Here's how the part is built. I have some questions about the finished solid (model axes, mm). Give positions to 0.01 mm unless a question says otherwise; leave off trailing zeros. Loops run counter-clockwise (first coordinate to the right, second up) from the corner with the lowest first, then second, coordinate; pieces in that order, holes last.
Q1. I'm going to push flat-ended pins straight in: P1, Ø5, axis at x = 81.5, z = 31, coming from the -Y side; P2, Ø8, axis at x = 22.5, y = -34, coming from the -Z side; P3, Ø8, axis at x = 86, y = -18, coming from the +Z side. Where does each tip first touch, or does it pass through?
Q2. I need wall thicknesses on probe 1 along X at (y, z) = (-5.5, 40); probe 2 along X at (y, z) = (-10.5, 32); probe 3 along X at (y, z) = (-2.5, 58). Which ranges of each line are inside material? Lowest first, please.
Q3. Suppose I cut it at D-D (x = 144). List the corners of the cut face in (y, z) for me.
Q4. Thinking about a two-plate mould opening in Z: for faces 1 (the face through (148, -50.8, 24)), 2 (the face through (99.35, -41.14, 39.4)), 3 (the face through (-53.17, -25.04, 13.87)), which applies, pulls with the +Z half, pulls with the -Z half, needs draft (parallel to the pull), parting line crosses it, or undercut?
Q5. Suppose I cut it at C-C (z = 44.5). List the corners of the cut face in (x, y) for me.
Q6. Suppose I cut it at B-B (y = -9.5). List the corners of the cut face in (x, z) for me (1 decimal).
Q7. Suppose I cut it at A-A (y = -35). List the corners of the cut face in (x, z) for me (1 decimal).
```python
from build123d import *
from build123d import SkipClean  # not in build123d's __all__

# Parameters (mm, degrees)
F0_R     = 17.4625
F1_DEPTH = 31.75
F2_DEPTH = 31.75
F0_R_2   = 25.4
F3_DEPTH = 50.8
F4_DEPTH = 12.7
F5_DEPTH = 50.8


with BuildPart() as f1:
    # F0 (on Front) → F1 (new body)
    with BuildSketch(Plane.XZ):
        with BuildLine():
            ThreePointArc((137.8952277792, 72.3404701197), (134.9898494581, 72.609247784), (132.0721238048, 72.6277311095))
            Line((132.0721238048, 72.6277311095), (137.8952277792, 72.3404701197))
        make_face()
        with BuildLine():
            Line((137.8952277792, 5.0155493856), (132.0808217973, 4.7279708331))
            ThreePointArc((132.0808217973, 4.7279708331), (134.9941960526, 4.7469864233), (137.8952277792, 5.0155493856))
        make_face()
        with BuildLine():
            Line((137.8952277792, 72.3404701197), (132.0721238048, 72.6277311095))
            ThreePointArc((132.0721238048, 72.6277311095), (99.3434793984, 38.6736578588), (132.0808217973, 4.7279708331))
            Line((132.0808217973, 4.7279708331), (137.8952277792, 5.0155493856))
            ThreePointArc((137.8952277792, 5.0155493856), (158.9060092226, 16.333410504), (167.2884791197, 38.6780097526))
            ThreePointArc((167.2884791197, 38.6780097526), (158.9060092226, 61.0226090013), (137.8952277792, 72.3404701197))
        make_face()
        with Locations((133.3159791197, 38.6780097526)):
            Circle(F0_R, mode=Mode.SUBTRACT)
    extrude(amount=F1_DEPTH)

    # F0 (on Front) → F2 (join)
    with BuildSketch(Plane.XZ):
        with BuildLine():
            ThreePointArc((-42.8278144375, 81.2557634421), (-15.6881628684, 67.2156297522), (-4.7965205083, 38.6664061547))
            ThreePointArc((-4.7965205083, 38.6664061547), (-15.6881628684, 10.1171825573), (-42.8278144375, -3.9229511326))
            Line((-42.8278144375, -3.9229511326), (132.0808217973, 4.7279708331))
            ThreePointArc((132.0808217973, 4.7279708331), (99.3434793984, 38.6736578588), (132.0721238048, 72.6277311095))
            Line((132.0721238048, 72.6277311095), (-42.8278144375, 81.2557634421))
        make_face()
    extrude(amount=F2_DEPTH)

    # F0 (on Front) → F3 (join)
    with BuildSketch(Plane.XZ):
        with BuildLine():
            ThreePointArc((-42.8278144375, -3.9229511326), (-15.6881628684, 10.1171825573), (-4.7965205083, 38.6664061547))
            ThreePointArc((-4.7965205083, 38.6664061547), (-15.6881628684, 67.2156297522), (-42.8278144375, 81.2557634421))
            ThreePointArc((-42.8278144375, 81.2557634421), (-90.5215205083, 38.6664061547), (-42.8278144375, -3.9229511326))
        make_face()
        with Locations((-47.6590205083, 38.6664061547)):
            Circle(F0_R_2, mode=Mode.SUBTRACT)
    extrude(amount=F3_DEPTH)

    # F0 (on Front) → F4 (cut)
    with BuildSketch(Plane.XZ):
        with BuildLine():
            ThreePointArc((-42.8278144375, 81.2557634421), (-15.6881628684, 67.2156297522), (-4.7965205083, 38.6664061547))
            ThreePointArc((-4.7965205083, 38.6664061547), (-15.6881628684, 10.1171825573), (-42.8278144375, -3.9229511326))
            Line((-42.8278144375, -3.9229511326), (132.0808217973, 4.7279708331))
            ThreePointArc((132.0808217973, 4.7279708331), (99.3434793984, 38.6736578588), (132.0721238048, 72.6277311095))
            Line((132.0721238048, 72.6277311095), (-42.8278144375, 81.2557634421))
        make_face()
    with SkipClean():  # cleaning this boolean's faces spoils the solid; the shape is the same uncleaned
        extrude(amount=F4_DEPTH, mode=Mode.SUBTRACT)

    # F0 (on Front) → F5 (join)
    with BuildSketch(Plane.XZ):
        with BuildLine():
            Line((137.8952277792, 72.3404701197), (132.0721238048, 72.6277311095))
            ThreePointArc((132.0721238048, 72.6277311095), (99.3434793984, 38.6736578588), (132.0808217973, 4.7279708331))
            Line((132.0808217973, 4.7279708331), (137.8952277792, 5.0155493856))
            ThreePointArc((137.8952277792, 5.0155493856), (158.9060092226, 16.333410504), (167.2884791197, 38.6780097526))
            ThreePointArc((167.2884791197, 38.6780097526), (158.9060092226, 61.0226090013), (137.8952277792, 72.3404701197))
        make_face()
        with Locations((133.3159791197, 38.6780097526)):
            Circle(F0_R, mode=Mode.SUBTRACT)
    with SkipClean():  # cleaning this boolean's faces spoils the solid; the shape is the same uncleaned
        extrude(amount=F5_DEPTH)


solid = f1.part
```
Solutions:
1. P1: stops at y = -31.75
1. P2: stops at z = -0.86
1. P3: stops at z = 75.1
2. probe 1: x = -90.5 to -73.02, -22.29 to -4.82, 99.37 to 115.9, 150.73 to 167.26
2. probe 2: x = -90 to -72.17, -23.15 to -5.32, 100.01 to 117.18, 149.45 to 166.63
2. probe 3: x = -85.91 to -64.13, -31.19 to -9.4, 105.37 to 161.26
3. outline: (-50.8, 6.43) - (0, 6.43) - (0, 24.87) - (-50.8, 24.87) - close; (-50.8, 52.49) - (0, 52.49) - (0, 70.93) - (-50.8, 70.93) - close
4. face 1: needs draft
4. face 2: parting line crosses it
4. face 3: undercut
5. outline: (-90.12, -50.8) - (-72.38, -50.8) - (-72.38, 0) - (-90.12, 0) - close; (-22.94, -50.8) - (-5.2, -50.8) - (-5.2, -31.75) - (99.85, -31.75) - (99.85, -50.8) - (116.85, -50.8) - (116.85, 0) - (99.85, 0) - (99.85, -12.7) - (-5.2, -12.7) - (-5.2, 0) - (-22.94, 0) - close; (149.78, -50.8) - (166.79, -50.8) - (166.79, 0) - (149.78, 0) - close
6. outline: circle Ø85.7 at (-47.7, 38.7); circle Ø67.9 at (133.3, 38.7); hole circle Ø50.8 at (-47.7, 38.7); hole circle Ø34.9 at (133.3, 38.7)
7. outline: circle Ø85.7 at (-47.7, 38.7); (132.1, 4.7) - (137.9, 5) arc R34 ccw to (137.9, 72.3) - (132.1, 72.6) arc R34 ccw to start; hole circle Ø50.8 at (-47.7, 38.7); hole circle Ø34.9 at (133.3, 38.7)
